Work out the finished part from the listing and answer in its coordinate system (mm). A direction names the side the tool comes from. Round coordinates to 2 decimals unless told otherwise and drop trailing zeros. Write each loop counter-clockwise with the first axis right and the second up, starting at its lowest first coordinate (ties: lowest second). Pieces come first, ordered by that corner, then holes. Notation, with made-up numbers: (-4, 67.5) - (55, 67.5) arc R28 cw to (55, 94.5) - close; hole circle Ø9 at (-35, 70.25). An arc over 180 degrees is marked (long way). Answer as a JSON object with one key per item and string values.
```python
from build123d import *

# Parameters (mm, degrees)
F0_W     = 88.9
F0_H     = 927.1
F1_DEPTH = 38.1
F2_W     = 1524
F2_H     = 139.7
F3_DEPTH = 19.05
F4_W     = 1703.7423849106
F4_H     = 635.3735253215
F5_DEPTH = 152.4


with BuildPart() as f1:
    # F0 (on Front) → F1 (new body)
    with BuildSketch(Plane.XZ):
        with Locations((44.45, 463.55)):
            Rectangle(F0_W, F0_H)
    extrude(amount=F1_DEPTH)

    # F2 (on face) → F3 (join)
    with BuildSketch(Plane(origin=(0, 0, 0), x_dir=(-1, 0, 0), z_dir=(0, 1, 0))):
        with Locations((36.5120689366, 222.25)):
            Rectangle(F2_W, F2_H)
        with Locations((36.5120689366, 539.75)):
            Rectangle(F2_W, F2_H)
        with Locations((36.5120689366, 857.25)):
            Rectangle(F2_W, F2_H)
    extrude(amount=F3_DEPTH)

    # F4 (on Top) → F5 (join)
    with BuildSketch(Plane.XY):
        with Locations((-92.205286026, 317.6867626607)):
            Rectangle(F4_W, F4_H)
    extrude(amount=F5_DEPTH)


solid = f1.part
```
Item 1: Determine the mould class of faces 6 (the flat face through (759.666, 313, 75)), 7 (the flat face through (-104, 303, 0)), 8 (the flat face through (-40, 3, 927.1)), 9 (the flat face through (44, 0, 700)) for opening direction Z: pulls with the +Z half, pulls with the -Z half, needs draft (parallel to the pull), parting line crosses it, or undercut.
Results found:
{"face 6": "needs draft", "face 7": "pulls with the -Z half", "face 8": "pulls with the +Z half", "face 9": "undercut"}
Item 2: A cutting plane is placed at A-A (x = -196). Write down the section's boundary in (y, z), and give its area (3 significant figures).
Results found:
{"outline": "(0, 0) - (635.37, 0) - (635.37, 152.4) - (19.05, 152.4) - (19.05, 292.1) - (0, 292.1) - close; (0, 469.9) - (19.05, 469.9) - (19.05, 609.6) - (0, 609.6) - close; (0, 787.4) - (19.05, 787.4) - (19.05, 927.1) - (0, 927.1) - close", "area": "105,000 mm²"}
Item 3: Consider line 1 along Z through (x, y) = (-486, 142.5); line 2 along Y through (x, z) = (-682.5, 537); line 3 along Y through (x, z) = (-593, 102). Determine where each line is inside the solid, lowest interval first.
Results found:
{"line 1": "0 to 152.4", "line 2": "0 to 19.05", "line 3": "0 to 635.37"}
Item 4: A cutting plane is placed at B-B (z = 574). Write down the section's boundary in (x, y), and give its area (3 significant figures).
Results found:
{"outline": "(-798.51, 0) - (0, 0) - (0, -38.1) - (88.9, -38.1) - (88.9, 0) - (725.49, 0) - (725.49, 19.05) - (-798.51, 19.05) - close", "area": "32,400 mm²"}
Item 5: A cutting plane is placed at D-D (z = 675). Write down the section's boundary in (x, y).
Results found:
{"outline": "(0, -38.1) - (88.9, -38.1) - (88.9, 0) - (0, 0) - close"}
Item 6: Each of these flat-tipped pins is pushed along its axis until it touches: P1, Ø21, axis at y = 5, z = 505.5, coming from the -X side; P2, Ø9.5, axis at y = 13.5, z = 868, coming from the +X side; P3, Ø19, axis at y = -23.5, z = 595, coming from the +X side. Where does it stop, or does it pass through?
Results found:
{"P1": "x = -798.51", "P2": "x = 725.49", "P3": "x = 88.9"}
Item 7: For faces 1 (the flat face through (-944.076, 313, 75)), 2 (the flat face through (412, 0, 858)), 3 (the flat face through (-26, 19.05, 223)), 4 (the flat face through (44, 0, 382)), 5 (the flat face through (0, -19, 457)), determine the directions among +Z, -Z, +X, -X, +Y, -Y from which every point of the face is accessible in a straight line to the end or side of a thin tool.
Results found:
{"face 1": "+Z, -Z, -X, +Y, -Y", "face 2": "+Z, -Z, +X, -Y", "face 3": "+Z, +X, -X, +Y", "face 4": "+X, -X, +Y", "face 5": "+Z, -Z, -X, -Y"}
Item 8: A cutting plane is placed at C-C (y = 352). Write down the section's boundary in (x, z).
Results found:
{"outline": "(-944.08, 0) - (759.67, 0) - (759.67, 152.4) - (-944.08, 152.4) - close"}
